```python
from build123d import *

# Parameters (mm, degrees)
F1_DEPTH = 3.175


with BuildPart() as f1:
    # F0 (on Front) → F1 (new body)
    with BuildSketch(Plane.XZ):
        with BuildLine():
            Line((-11.770303, 14.329202), (-12.722803, 14.329202))
            ThreePointArc((-12.722803, 14.329202), (-13.754507, 13.901856), (-14.181852, 12.870152))
            Line((-14.181852, 12.870152), (-14.181852, -13.164848))
            ThreePointArc((-14.181852, -13.164848), (-13.754507, -14.196552), (-12.722803, -14.623898))
            Line((-12.722803, -14.623898), (-11.770303, -14.623898))
            ThreePointArc((-11.770303, -14.623898), (-9.883423, -15.405469), (-9.101852, -17.292348))
            Line((-9.101852, -17.292348), (-9.101852, -18.244848))
            ThreePointArc((-9.101852, -18.244848), (-8.674507, -19.276552), (-7.642803, -19.703898))
            Line((-7.642803, -19.703898), (8.232197, -19.703898))
            ThreePointArc((8.232197, -19.703898), (9.263901, -19.276552), (9.691247, -18.244848))
            Line((9.691247, -18.244848), (9.691247, -17.292348))
            ThreePointArc((9.691247, -17.292348), (10.472818, -15.405469), (12.359697, -14.623898))
            Line((12.359697, -14.623898), (13.312197, -14.623898))
            ThreePointArc((13.312197, -14.623898), (14.343901, -14.196552), (14.771247, -13.164848))
            Line((14.771247, -13.164848), (14.771247, 12.870152))
            ThreePointArc((14.771247, 12.870152), (14.343901, 13.901856), (13.312197, 14.329202))
            Line((13.312197, 14.329202), (12.359697, 14.329202))
            ThreePointArc((12.359697, 14.329202), (10.472818, 15.110773), (9.691247, 16.997652))
            Line((9.691247, 16.997652), (9.691247, 17.950152))
            ThreePointArc((9.691247, 17.950152), (9.263901, 18.981856), (8.232197, 19.409202))
            Line((8.232197, 19.409202), (-7.642803, 19.409202))
            ThreePointArc((-7.642803, 19.409202), (-8.674507, 18.981856), (-9.101852, 17.950152))
            Line((-9.101852, 17.950152), (-9.101852, 16.997652))
            ThreePointArc((-9.101852, 16.997652), (-9.883423, 15.110773), (-11.770303, 14.329202))
        make_face()
    extrude(amount=F1_DEPTH)


solid = f1.part
```
Input: part model. Units: mm. Frame: model coordinates. A direction names the side the tool comes from. Coordinates: 2 decimals unless noted, no trailing zeros. Loops run counter-clockwise (first coordinate to the right, second up) from the corner with the lowest first, then second, coordinate; pieces in that order, holes last.
Q1. Section A-A, the plane y = -0.9. Return the cut outline in (x, z), and give its area (3 significant figures).
Results are:
outline: (-14.18, -13.16) arc R1.46 ccw to (-12.72, -14.62) - (-11.77, -14.62) arc R2.67 cw to (-9.1, -17.29) - (-9.1, -18.24) arc R1.46 ccw to (-7.64, -19.7) - (8.23, -19.7) arc R1.46 ccw to (9.69, -18.24) - (9.69, -17.29) arc R2.67 cw to (12.36, -14.62) - (13.31, -14.62) arc R1.46 ccw to (14.77, -13.16) - (14.77, 12.87) arc R1.46 ccw to (13.31, 14.33) - (12.36, 14.33) arc R2.67 cw to (9.69, 17) - (9.69, 17.95) arc R1.46 ccw to (8.23, 19.41) - (-7.64, 19.41) arc R1.46 ccw to (-9.1, 17.95) - (-9.1, 17) arc R2.67 cw to (-11.77, 14.33) - (-12.72, 14.33) arc R1.46 ccw to (-14.18, 12.87) - close
area: 1,030 mm2
Q2. Line query: line 1 along Z through (x, y) = (-12.75, -0.65); line 2 along X through (y, z) = (-2.4, -17.5); line 3 along Z through (x, y) = (10.25, -1.3). Output: solid intervals per line, ascending.
Results are:
line 1: z = -14.62 to 14.33
line 2: x = -9.1 to 9.69
line 3: z = -15.66 to 15.36
Q3. Contact query for flat-ended pins moving along their axis: pin 1 (0.8 mm diameter, centred on y = -1, z = -18, fed in from +X); pin 2 (1 mm diameter, centred on y = -1.5, z = 17.5, fed in from -X); pin 3 (3 mm diameter, centred on x = 3, z = 0, fed in from +Y); pin 4 (0.5 mm diameter, centred on x = 13, y = -2, fed in from +Z). Output: stop coordinate, or through.
Results are:
pin 1: stops at x = 9.69
pin 2: stops at x = -9.1
pin 3: stops at y = 0
pin 4: stops at z = 14.33
Q4. Section C-C, the plane z = -16.5. Return the cut outline in (x, y) (3 decimals).
Results are:
outline: (-9.222, -3.175) - (9.812, -3.175) - (9.812, 0) - (-9.222, 0) - close
Q5. Set-up query: faces 1 (the flat face through (-12, -2, -14.624)), 2 (the flat face through (-9.102, -1.6, 17.5)), 3 (the flat face through (9.691, -1.6, 17.5)). Return all of +Z, -Z, +X, -X, +Y, -Y with unobstructed straight access to the full face (end or side cutting, diameter ignored); none if empty.
Results are:
face 1: -Z, -X, +Y, -Y
face 2: +Z, -X, +Y, -Y
face 3: +Z, +X, +Y, -Y
Q6. Section B-B, the plane x = -10.5. Return the cut outline in (y, z) (3 decimals).
Results are:
outline: (-3.175, -14.946) - (0, -14.946) - (0, 14.651) - (-3.175, 14.651) - close
